Verification items for the finished model (mm, model axes). A direction names the side the tool comes from. Coordinates: 2 decimals unless noted, no trailing zeros. Write each loop counter-clockwise with the first axis right and the second up, starting at its lowest first coordinate (ties: lowest second). Pieces come first, ordered by that corner, then holes. Notation, with made-up numbers: (7, 68) -> (41, 68) arc R24 ccw to (41, 87) -> close; hole circle Ø11 at (-34, 26). An arc over 180 degrees is marked (long way). Write item = value, one per line. Start each with the question number.
(1) Set-up check for faces 5 (the face through (-46.038, 18, -1)), 6 (the face through (50.8, 14, -1)): record each of +Z, -Z, +X, -X, +Y, -Y from which the full face is reachable in a straight line by a thin tool's end or side.
(2) Section check A-A (x = 0). Record the cut outline in (y, z), plus the area to 3 significant figures.
(3) Section check D-D (x = -31.5). Record the cut outline in (y, z).
(4) Section check C-C (z = 9). Record the cut outline in (x, y).
(5) Mould release check, pull along Z, two halves, no side actions. Record for faces 1 (the face through (0, 4, -74.254)), 2 (the face through (-23, 0, -18)), 3 (the face through (0, 4, 74.254)), 4 (the face through (33.165, 2.415, 58.575)): released by +Z, released by -Z, zero draft, split by the parting line, or undercut.
(6) Gauge pin test, flat end, axial feed: pin 1 Ø7.5 at (x, z) = (33.02, -61.87) entering from +Y. Record the tip position at first contact, or that the pin passes through.
(7) Section check B-B (y = 18). Record the cut outline in (x, z).
(8) Material ranges on probe 1 along X at (y, z) = (9, -46); probe 2 along X at (y, z) = (4, 62); probe 3 along Y at (x, z) = (-19.5, 45), recorded low to high. Write a range as [from, to].
```python
from build123d import *

# Parameters (mm, degrees)
EXTRUDE_THIN1_DEPTH  = 74.25436
FILLET1_RADIUS       = 2.38125
FILLET1_LENGTH       = 74.25436
FILLET2_R            = 2.54
MIRROR1_START        = -74.25436
MIRROR1_DEPTH        = 148.50872
M6_CLEARANCE_HOLE1_D = 6.6
SKETCH11_R           = 34.925
CUT_EXTRUDE4_DEPTH   = 94.929096319


# Read off the part's stored shape, not the designer's step: Mirror1
with BuildPart() as part:
    # Sketch4 → Extrude-Thin1 (new body)
    with BuildSketch(Plane.XY):
        Polygon((0, 0), (-50.8, 0), (-50.8, 31.75), (-46.0375, 31.75), (-46.0375, 4.7625), (0, 4.7625), align=None)
    extrude(amount=EXTRUDE_THIN1_DEPTH)

    # Fillet1: full round fillet: the end face becomes a half cylinder, R = half its width
    fillet1_face = Plane((-48.41875, 31.75, 37.12718), x_dir=(0, 0, -1), z_dir=(0, 1, 0))  # on the end face: x along it, z out of the body
    fillet1_slab = fillet1_face.offset(-FILLET1_RADIUS / 2) * Box(FILLET1_LENGTH, 2 * FILLET1_RADIUS, FILLET1_RADIUS, mode=Mode.PRIVATE)  # the body's end, R deep
    fillet1_round = Plane((-48.41875, 29.36875, 37.12718), x_dir=(0, 1, 0), z_dir=(0, 0, -1)) * Cylinder(FILLET1_RADIUS, FILLET1_LENGTH, mode=Mode.PRIVATE)  # its axis R under the face
    add(fillet1_slab - fillet1_round, mode=Mode.SUBTRACT)

    # Fillet2
    fillet2_edges = [part.edges().sort_by_distance(p)[0] for p in [
        (-46.0375, 4.7625, 37.12718),
    ]]
    fillet(fillet2_edges, radius=FILLET2_R)

    # Mirror1 outline → Mirror1 (add)
    with BuildSketch(Plane.XY.offset(MIRROR1_START)):
        with BuildLine():
            ThreePointArc((-46.0375, 29.36875), (-48.41875, 31.75), (-50.8, 29.36875))
            Line((-50.8, 29.36875), (-50.8, 0))
            Line((-50.8, 0), (50.8, 0))
            Line((50.8, 0), (50.8, 29.36875))
            ThreePointArc((50.8, 29.36875), (48.41875, 31.75), (46.0375, 29.36875))
            Line((46.0375, 29.36875), (46.0375, 7.3025))
            ThreePointArc((46.0375, 7.3025), (45.293551224, 5.506448776), (43.4975, 4.7625))
            Line((43.4975, 4.7625), (-43.4975, 4.7625))
            ThreePointArc((-43.4975, 4.7625), (-45.293551224, 5.506448776), (-46.0375, 7.3025))
            Line((-46.0375, 7.3025), (-46.0375, 29.36875))
        make_face()
    extrude(amount=MIRROR1_DEPTH)

    # M6 Clearance Hole1 (through all)
    with Locations(Plane(origin=(-33.02, 0, 61.87186), x_dir=(0, 0, -1), z_dir=(0, -1, 0))):
        with Locations((0, 0), (0, 66.04), (123.74372, 0), (123.74372, 66.04)):
            Hole(M6_CLEARANCE_HOLE1_D / 2)

    # Sketch11 → Cut-Extrude4 (cut, through all)
    with BuildSketch(Plane(origin=(0, 4.7625, 0), x_dir=(1, 0, 0), z_dir=(0, 1, 0))):
        with Locations(Location((0, -10.75436, 0), (0, 0, 270))):
            Circle(SKETCH11_R)
    extrude(amount=-CUT_EXTRUDE4_DEPTH, mode=Mode.SUBTRACT)


solid = part.part
```
Response:
q1.face_5 = +Z, -Z, +Y
q1.face_6 = +Z, -Z, +X, +Y, -Y
q2.outline = (0, -74.25) -> (4.76, -74.25) -> (4.76, -24.17) -> (0, -24.17) -> close; (0, 45.68) -> (4.76, 45.68) -> (4.76, 74.25) -> (0, 74.25) -> close
q2.area = 375 mm2
q3.outline = (0, -74.25) -> (4.76, -74.25) -> (4.76, -64.8) -> (0, -64.8) -> close; (0, -58.94) -> (4.76, -58.94) -> (4.76, -4.33) -> (0, -4.33) -> close; (0, 25.84) -> (4.76, 25.84) -> (4.76, 58.94) -> (0, 58.94) -> close; (0, 64.8) -> (4.76, 64.8) -> (4.76, 74.25) -> (0, 74.25) -> close
q4.outline = (-50.8, 0) -> (-34.88, 0) -> (-34.88, 4.76) -> (-43.5, 4.76) arc R2.54 cw to (-46.04, 7.3) -> (-46.04, 29.37) arc R2.38 ccw to (-50.8, 29.37) -> close; (34.88, 0) -> (50.8, 0) -> (50.8, 29.37) arc R2.38 ccw to (46.04, 29.37) -> (46.04, 7.3) arc R2.54 cw to (43.5, 4.76) -> (34.88, 4.76) -> close
q5.face_1 = released by -Z
q5.face_2 = zero draft
q5.face_3 = released by +Z
q5.face_4 = undercut
q6.pin_1 = 4.76
q7.outline = (-50.8, -74.25) -> (-46.04, -74.25) -> (-46.04, 74.25) -> (-50.8, 74.25) -> close; (46.04, -74.25) -> (50.8, -74.25) -> (50.8, 74.25) -> (46.04, 74.25) -> close
q8.probe_1 = [-50.8, -46.04], [46.04, 50.8]
q8.probe_2 = [-50.8, -36.32], [-29.72, 29.72], [36.32, 50.8]
q8.probe_3 = [0, 4.76]
